Design review of the part built by this model. Coordinates are the model's own, in mm. Face numbers are marked on the shaded views. Coordinates: 2 decimals unless noted, no trailing zeros. Order: outer loops, then holes, each group sorted by start corner. A loop starts at its lowest first (then second) coordinate and runs counter-clockwise, first axis right, second up. Notation, with made-up numbers: (-30, 23) - (-26, 23) arc R17 ccw to (-26, 48) - close; hole circle Ø5 at (-1.5, 54.5). An arc over 180 degrees is marked (long way). Write item = value, one per line. Start each with the question number.
```python
from build123d import *

# Parameters (mm, degrees)
SKETCH2_R           = 9.525
SKETCH2_R_2         = 1.4224
SKETCH2_R_3         = 2.5
BOSS_EXTRUDE1_DEPTH = 5.08
CUT_EXTRUDE1_REACH  = 15.47
SKETCH7_R           = 1.4224


with BuildPart() as part:
    # Sketch2 → Boss-Extrude1 (new body)
    with BuildSketch(Plane(origin=(0, 0, 0), x_dir=(1, 0, 0), z_dir=(0, 1, 0))):
        Circle(SKETCH2_R)
        with Locations((0, 6.35)):
            Circle(SKETCH2_R_2, mode=Mode.SUBTRACT)
        with Locations((6.35, 0)):
            Circle(SKETCH2_R_2, mode=Mode.SUBTRACT)
        with Locations((0, -6.35)):
            Circle(SKETCH2_R_2, mode=Mode.SUBTRACT)
        with Locations((-6.35, 0)):
            Circle(SKETCH2_R_2, mode=Mode.SUBTRACT)
        Circle(SKETCH2_R_3, mode=Mode.SUBTRACT)
    extrude(amount=BOSS_EXTRUDE1_DEPTH)

    # Sketch7 → Cut-Extrude1 (cut, up to next)
    with BuildSketch(Plane(origin=(0, 0, 0), x_dir=(0.707106781, 0, -0.707106781), z_dir=(0.707106781, 0, 0.707106781)), mode=Mode.PRIVATE) as cut_extrude1_sk1:
        with Locations((0, 2.54)):
            Circle(SKETCH7_R)
    cut_extrude1_tool1 = extrude(cut_extrude1_sk1.sketch, amount=-CUT_EXTRUDE1_REACH, mode=Mode.PRIVATE) & part.part
    add(cut_extrude1_tool1.solids().sort_by_distance((0, 2.54, 0))[0], mode=Mode.SUBTRACT)


solid = part.part
```
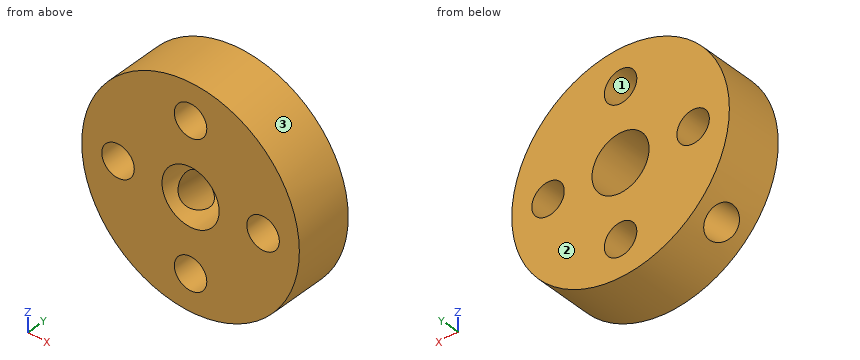
Item 1: Add section B-B on x = 0. Give the boundary of the cut face in (y, z) (3 decimals).
Item 2: For P1, Ø3, axis at y = 1, z = -6, coming from the +X side (3 decimals); P2, Ø1.7, axis at x = -6.35, z = 0, coming from the +Y side; P3, Ø1.5, axis at y = 4.5, z = -3, coming from the -X side; P4, Ø1, axis at x = -3, y = 4.5, coming from the -Z side, all flat-tipped, find the tip position at first contact; note any pin that passes through.
Item 3: Add section D-D on z = 6.35. Give the boundary of the cut face in (x, y).
Item 4: Add section A-A on z = 0. Give the boundary of the cut face in (x, y) (3 decimals).
Item 5: For line 1 (Z direction, x = 0, y = 1.35) (3 decimals); line 2 (Z direction, x = -0.5, y = 4.3), list the stretches that pass through material, from the lowest coordinate up.
Item 6: Mouldability with a two-part tool opening along Z and no side actions: class the marked faces 1, 2 and 3 as +Z half, -Z half, draft (parallel to the pull), parting line (faces both ways), or undercut.
Item 7: Add section C-C on y = 2.3. Give the boundary of the cut face in (x, z) (3 decimals), plus the area to 3 significant figures.
Worked out:
q1.outline = (0, -9.525) - (5.08, -9.525) - (5.08, -7.772) - (0, -7.772) - close; (0, -4.928) - (5.08, -4.928) - (5.08, -2.5) - (0, -2.5) - close; (0, 2.5) - (5.08, 2.5) - (5.08, 4.928) - (0, 4.928) - close; (0, 7.772) - (5.08, 7.772) - (5.08, 9.525) - (0, 9.525) - close
q2.P1 = 8.395
q2.P2 = through
q2.P3 = -9.26
q2.P4 = -9.19
q3.outline = (-7.1, 0) - (-1.42, 0) - (-1.42, 5.08) - (-7.1, 5.08) - close; (1.42, 0) - (7.1, 0) - (7.1, 5.08) - (1.42, 5.08) - close
q4.outline = (-9.525, 0) - (-7.772, 0) - (-7.772, 5.08) - (-9.525, 5.08) - close; (-4.928, 0) - (-2.5, 0) - (-2.5, 5.08) - (-4.928, 5.08) - close; (2.5, 0) - (4.928, 0) - (4.928, 5.08) - (2.5, 5.08) - close; (7.772, 0) - (9.525, 0) - (9.525, 5.08) - (7.772, 5.08) - close
q5.line_1 = -9.525 to -7.772, -4.928 to -2.5, 2.5 to 4.928, 7.772 to 9.525
q5.line_2 = -9.51 to -7.68, -5.02 to -2.45, 2.45 to 5.02, 7.68 to 9.51
q6.face_1 = undercut
q6.face_2 = draft
q6.face_3 = parting line
q7.outline = (-7.653, -5.67) - (-2.455, -0.472) arc R2.5 cw (long way) to (-0.472, -2.455) - (-5.67, -7.653) arc R9.525 ccw (long way) to start; hole circle Ø2.845 at (-6.35, 0); hole circle Ø2.845 at (0, -6.35); hole circle Ø2.845 at (0, 6.35); hole circle Ø2.845 at (6.35, 0)
q7.area = 220 mm2
